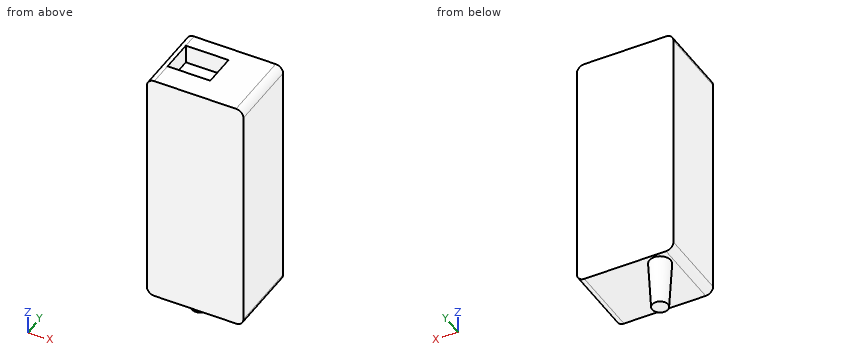
Autodesk Inventor part; units mm, degrees
ref_plane "Work Plane1" through (-4, 0, -155) normal (0, 0, -1) x (-1, 0, 0)
ref_plane "YZ Plane" through (0, 0, 0) normal (1, 0, 0) x (0, 1, 0)
ref_plane "XZ Plane" through (0, 0, 0) normal (0, 1, 0) x (-1, 0, 0)
sketch "Sketch1" plane through (0, 0, 0) normal (0, 1, 0) x (-1, 0, 0)
  line L0 (0, 0) -> (52, 0)
  line L1 (52, 0) -> (52, -129)
  line L2 (52, -129) -> (0, -129)
  line L3 (0, -129) -> (0, 0)
  dimension "d0" = 52
  dimension "d1" = 129
extrude "Extrusion1" add sketch "Sketch1" along normal blind 39
fillet "Fillet1" radius 4 4 edges at (0, 19.5, 0) (0, 19.5, -129) (-52, 19.5, 0) (-52, 19.5, -129)
sketch "Sketch2" plane through (-48, 0, 0) normal (0, 0, 1) x (1, 0, 0)
  line L0 (44, 39) -> (0, 39)
  line L1 (0, 39) -> (0, 31)
  line L2 (0, 39) -> (0, 0)
  line L3 (0, 31) -> (23, 31)
  line L4 (23, 31) -> (23, 13)
  line L5 (23, 13) -> (0, 13)
  line L6 (0, 13) -> (0, 31)
  point P0 (48, 0)
  dimension "d5" = 8
  dimension "d6" = 23
  dimension "d7" = 18
extrude "Extrusion2" cut sketch "Sketch2" against normal blind 10
sketch "Sketch3" plane through (-4, 0, -129) normal (0, 0, -1) x (-1, 0, 0)
  line L0 (0, 39) -> (44, 39)
  line L1 (44, 39) -> (44, 36)
  line L2 (44, 39) -> (44, 0)
  line L3 (44, 36) -> (41, 36)
  line L4 (41, 36) -> (36.9695, 31.9695)
  line L5 (41, 36) -> (46.7, 36) construction
  circle A0 centre (36.9695, 31.9695) radius 5.7
  point P0 (-4, 0)
  dimension "d10" = 3
  dimension "d11" = 3
  dimension "d12" = 5.7
  dimension "d13" = 135
ref_plane "Work Plane1" through (-4, 0, -155) normal (0, 0, -1) x (-1, 0, 0)
sketch "Sketch4" plane through (-4, 0, -155) normal (0, 0, -1) x (-1, 0, 0)
  line L0 (0, 39) -> (44, 39)
  line L1 (44, 39) -> (44, 36)
  line L2 (44, 39) -> (44, 0)
  line L3 (44, 36) -> (41, 36)
  line L4 (41, 36) -> (36.9695, 31.9695)
  line L5 (41, 36) -> (46.7, 36) construction
  circle A0 centre (36.9695, 31.9695) radius 4.25
  point P0 (-4, 0)
  dimension "d15" = 3
  dimension "d16" = 3
  dimension "d17" = 5.7
  dimension "d18" = 135
  dimension "d19" = 8.5
loft "Loft1" add profiles "Sketch3", "Sketch4"
properties part number "NucPower"
Source: CAD feature listing. Evaluate the final solid. Frame: model axes, mm. Coordinates: 2 decimals unless noted, no trailing zeros. Loops run counter-clockwise (first coordinate to the right, second up) from the corner with the lowest first, then second, coordinate; pieces in that order, holes last. Notation, with made-up numbers: (26, 26.25) -> (80, 26.25) arc R23 cw to (80, 39.25) -> close; hole circle Ø7 at (24.25, 6). An arc over 180 degrees is marked (long way). One line per item, written item: value. Start each with the question number.
Q1. Contact query for flat-ended pins moving along their axis: P1, Ø4, axis at x = -39.5, y = 27.5, coming from the -Z side; P2, Ø8, axis at x = -12.5, y = 16, coming from the -Z side; P3, Ø5.5, axis at x = -32, y = 25.5, coming from the +Z side. Output: stop coordinate, or through.
Q2. Section query B-B, the plane z = -8.5. Return the cut outline in (x, y).
Q3. Section query A-A, the plane y = 4. Return the cut outline in (x, z).
Q4. Line query: line 1 along X through (y, z) = (17, -7); line 2 along Z through (x, y) = (-47, 35.5); line 3 along Z through (x, y) = (-3, 14.5). Output: solid intervals per line, ascending.
Q5. Section query C-C, the plane x = -20. Return the cut outline in (y, z).
Q6. Section query D-D, the plane y = 20. Return the cut outline in (x, z), and give its area (3 significant figures).
Results:
1. P1: z = -155
1. P2: z = -129
1. P3: z = -10
2. outline: (-52, 0) -> (0, 0) -> (0, 39) -> (-52, 39) -> close; hole (-48, 13) -> (-25, 13) -> (-25, 31) -> (-48, 31) -> close
3. outline: (-52, -125) arc R4 ccw to (-48, -129) -> (-4, -129) arc R4 ccw to (0, -125) -> (0, -4) arc R4 ccw to (-4, 0) -> (-48, 0) arc R4 ccw to (-52, -4) -> close
4. line 1: -52 to -48, -25 to 0
4. line 2: -129 to 0
4. line 3: -128.87 to -0.13
5. outline: (0, -129) -> (39, -129) -> (39, 0) -> (0, 0) -> close
6. outline: (-52, -125) arc R4 ccw to (-48, -129) -> (-4, -129) arc R4 ccw to (0, -125) -> (0, -4) arc R4 ccw to (-4, 0) -> (-25, 0) -> (-25, -10) -> (-48, -10) -> (-48, 0) arc R4 ccw to (-52, -4) -> close
6. area: 6,460 mm^2
